Autodesk Inventor part; units mm, degrees
ref_plane "YZ Plane" through (0, 0, 0) normal (1, 0, 0) x (0, 1, 0)
ref_plane "XZ Plane" through (0, 0, 0) normal (0, 1, 0) x (-1, 0, 0)
ref_plane "XY Plane" through (0, 0, 0) normal (0, 0, 1) x (1, 0, 0)
sketch "Sketch1" plane through (0, 0, 0) normal (0, 0, 1) x (1, 0, 0)
  line L0 (7.3323, 0) -> (3.6662, -6.35)
  line L1 (3.6662, -6.35) -> (-3.6662, -6.35)
  line L2 (-3.6662, -6.35) -> (-7.3323, 0)
  line L3 (-7.3323, 0) -> (-3.6662, 6.35)
  line L4 (-3.6662, 6.35) -> (3.6662, 6.35)
  line L5 (3.6662, 6.35) -> (7.3323, 0)
  point P0 (0, 0)
  point P1 (0, 0)
  dimension "d0" = 12.7
extrude "Extrusion1" add sketch "Sketch1" along normal blind 78.74
sketch "Sketch2" plane through (0, 0, 78.74) normal (0, 0, 1) x (1, 0, 0)
  circle A0 centre (0, 0) radius 5.842
  dimension "d7" = 11.684
extrude "Extrusion2" add sketch "Sketch2" along normal blind 1.0668
sketch "Sketch3" plane through (0, 0, 79.8068) normal (0, 0, 1) x (1, 0, 0)
  circle A0 centre (0, 0) radius 6.35
extrude "Extrusion3" add sketch "Sketch3" along normal blind 1.27
sketch "Sketch4" plane through (0, 0, 0) normal (0, 0, -1) x (-1, 0, 0)
  circle A0 centre (0, 0) radius 5.842
  circle A1 centre (0, 0) radius 6.35
  dimension "d8" = 11.684
extrude "Extrusion4" add sketch "Sketch4" along normal blind 1.0668 contours A0
sketch "Sketch5" plane through (0, 0, -1.0668) normal (0, 0, -1) x (-1, 0, 0)
  circle A0 centre (0, 0) radius 6.35
  dimension "d11" = 12.7
extrude "Extrusion5" add sketch "Sketch5" along normal blind 1.27
properties part number "CPS_007_HexShaftForCPS" material "Aluminum 6061"
Input: part model. Units: mm. Frame: model coordinates. A direction names the side the tool comes from. Round coordinates to 2 decimals unless told otherwise and drop trailing zeros. Write each loop counter-clockwise with the first axis right and the second up, starting at its lowest first coordinate (ties: lowest second). Pieces come first, ordered by that corner, then holes.
1) Cut plane B-B (y = 5). Return the cut outline in (x, z), then the cut area to 3 significant figures.
2) Cut plane A-A (z = 48). Return the cut outline in (x, y).
3) Draft query along Z for faces 4 (the flat face through (0, 6.35, 39)), 5 (the flat face through (6, 0, 78.74)), 6 (the flat face through (0, 0, 81.077)). Return one class per face: pulls with the +Z half, pulls with the -Z half, needs draft (parallel to the pull), parting line crosses it, or undercut.
4) Reachability of faces 1 (the cylindrical face through (1.38, 6.2, -1.69)), 2 (the cylindrical face through (-1.38, 6.2, 80.43)), 3 (the cylindrical face through (-1.266, 5.703, 79.266)) from +Z, -Z, +X, -X, +Y, -Y: full face, straight path, thin tool, end or side. Return the list, or none.
5) Cut plane C-C (y = -2.75). Return the cut outline in (x, z), then the cut area to 3 significant figures.
6) Contact query for flat-ended pins moving along their axis: P1, Ø6, axis at y = -5, z = 20, coming from the -X side; P2, Ø1.5, axis at y = -4.5, z = 42, coming from the +X side; P3, Ø1, axis at y = 1.5, z = 42, coming from the +X side. Output: stop coordinate, or through.
7) Ray query, L1, parallel to Z at x = 6, y = 0.5; L2, parallel to X at y = -1, z = 75; L3, parallel to X at y = 4.75, z = 14. Return the intervals inside material, ascending.
Geometry says:
1. outline: (-4.45, 0) - (-3.02, 0) - (-3.02, -1.07) - (-3.91, -1.07) - (-3.91, -2.34) - (3.91, -2.34) - (3.91, -1.07) - (3.02, -1.07) - (3.02, 0) - (4.45, 0) - (4.45, 78.74) - (3.02, 78.74) - (3.02, 79.81) - (3.91, 79.81) - (3.91, 81.08) - (-3.91, 81.08) - (-3.91, 79.81) - (-3.02, 79.81) - (-3.02, 78.74) - (-4.45, 78.74) - close
1. area: 733 mm2
2. outline: (-7.33, 0) - (-3.67, -6.35) - (3.67, -6.35) - (7.33, 0) - (3.67, 6.35) - (-3.67, 6.35) - close
3. face 4: needs draft
3. face 5: undercut
3. face 6: pulls with the +Z half
4. face 1: -Z
4. face 2: +Z
4. face 3: none
5. outline: (-5.74, 0) - (-5.15, 0) - (-5.15, -1.07) - (-5.72, -1.07) - (-5.72, -2.34) - (5.72, -2.34) - (5.72, -1.07) - (5.15, -1.07) - (5.15, 0) - (5.74, 0) - (5.74, 78.74) - (5.15, 78.74) - (5.15, 79.81) - (5.72, 79.81) - (5.72, 81.08) - (-5.72, 81.08) - (-5.72, 79.81) - (-5.15, 79.81) - (-5.15, 78.74) - (-5.74, 78.74) - close
5. area: 956 mm2
6. P1: stops at x = -6.18
6. P2: stops at x = 5.17
6. P3: stops at x = 6.75
7. L1: z = -2.34 to -1.07, 0 to 78.74, 79.81 to 81.08
7. L2: x = -6.75 to 6.75
7. L3: x = -4.59 to 4.59
